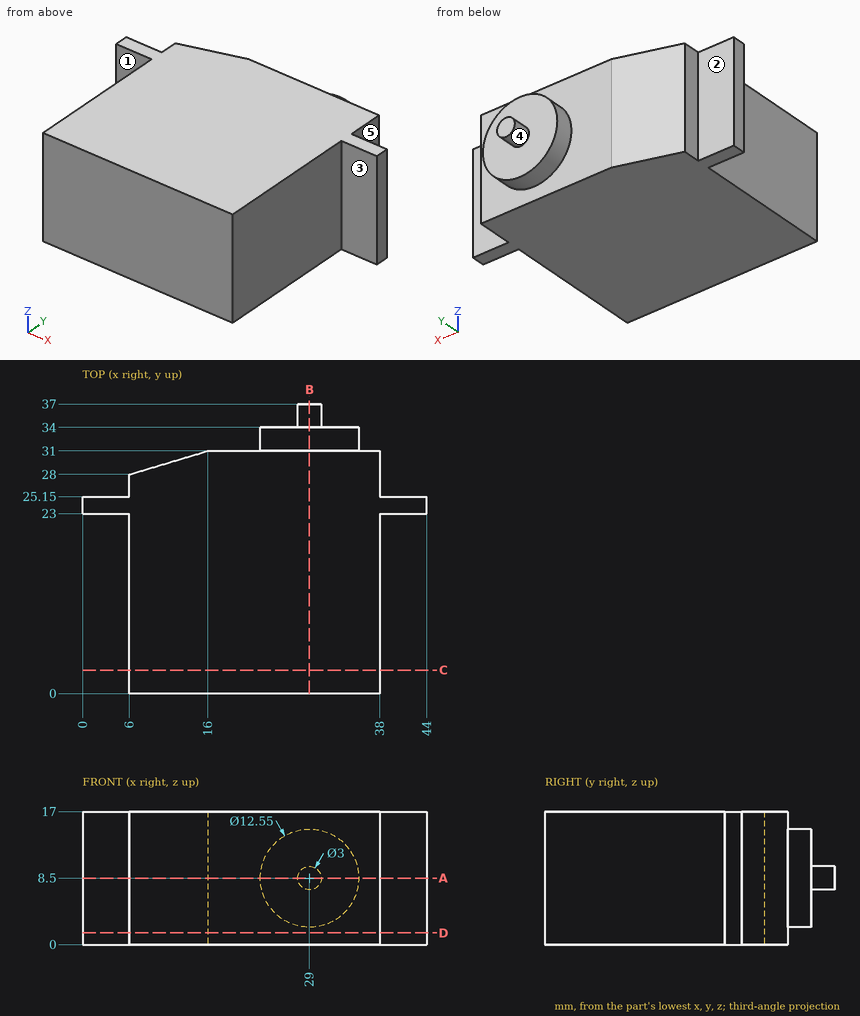
Geometry: see drawing. Coordinates: mm, zero at the bounding-box minimum. A direction names the side the tool comes from. Give positions to 0.01 mm unless a question says otherwise; leave off trailing zeros. Write each loop counter-clockwise with the first axis right and the second up, starting at its lowest first coordinate (ties: lowest second). Pieces come first, ordered by that corner, then holes. Notation, with made-up numbers: M 9.25,58 L 40.25,58 A20 ccw 40.25,88 Z; hole C 69,63 d3. An arc over 180 degrees is marked long. Answer in a Markdown table with one row per item. Add a question column.
(1) Section A-A on z = 8.5. Return loops of the section in (x, y) (3 decimals), and give its area (3 significant figures).
(2) Reachability of the marked faces 1, 2, 3, 4 and 5 from +Z, -Z, +X, -X, +Y, -Y: full face, straight path, thin tool, end or side. Return the list, or none.
(3) First-contact query: pin 1 (6.5 mm diameter, centred on x = 2.5, z = 9.5, fed in from +Y); pin 2 (8 mm diameter, centred on x = 18, y = 14.5, fed in from -Z); pin 3 (1.8 mm diameter, centred on y = 29.5, z = 6.5, fed in from +X); pin 4 (5 mm diameter, centred on x = 42, z = 5, fed in from -Y). Flat tips, straight axial feed; report the tip coordinate or a pass-through.
(4) Section B-B on x = 29. Return loops of the section in (y, z) (3 decimals).
(5) Section D-D on z = 1.5. Return loops of the section in (x, y).
(6) Ray query, line 1 (Y direction, x = 5, z = 7.25); line 2 (X direction, y = 7, z = 2.5); line 3 (Y direction, x = 31.5, z = 3.25). Return the intervals inside material, ascending.
(7) Section C-C on y = 3. Return loops of the section in (x, z).
Result set:
| question | item | result |
|---|---|---|
| 1 | outline | M 0,23 L 6,23 L 6,0 L 38,0 L 38,23 L 44,23 L 44,25.15 L 38,25.15 L 38,31 L 35.275,31 L 35.275,34 L 30.5,34 L 30.5,37 L 27.5,37 L 27.5,34 L 22.725,34 L 22.725,31 L 16,31 L 6,28 L 6,25.15 L 0,25.15 Z |
| 1 | area | 1,050 mm^2 |
| 2 | face 1 | +Z, -Z, -X, -Y |
| 2 | face 2 | +Z, -Z, -X, +Y |
| 2 | face 3 | +Z, -Z, +X, -Y |
| 2 | face 4 | +Y |
| 2 | face 5 | +Z, -Z, +X, +Y |
| 3 | pin 1 | stops at y = 25.15 |
| 3 | pin 2 | stops at z = 0 |
| 3 | pin 3 | stops at x = 38 |
| 3 | pin 4 | stops at y = 23 |
| 4 | outline | M 0,0 L 31,0 L 31,2.225 L 34,2.225 L 34,7 L 37,7 L 37,10 L 34,10 L 34,14.775 L 31,14.775 L 31,17 L 0,17 Z |
| 5 | outline | M 0,23 L 6,23 L 6,0 L 38,0 L 38,23 L 44,23 L 44,25.15 L 38,25.15 L 38,31 L 16,31 L 6,28 L 6,25.15 L 0,25.15 Z |
| 6 | line 1 | y = 23 to 25.15 |
| 6 | line 2 | x = 6 to 38 |
| 6 | line 3 | y = 0 to 34 |
| 7 | outline | M 6,0 L 38,0 L 38,17 L 6,17 Z |
